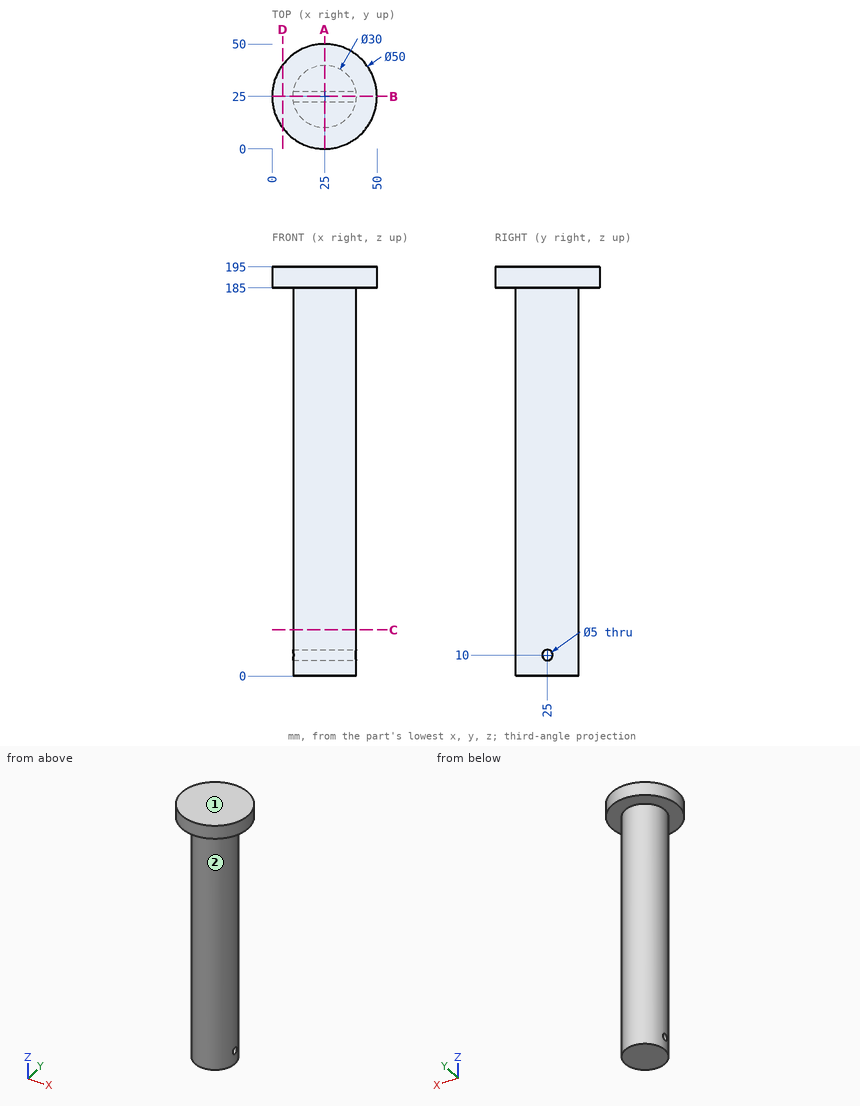
Check sheet for the drawn part. Datum: minimum x, y, z corner. Units: mm. Coordinates: 2 decimals unless noted, no trailing zeros. Order: outer loops, then holes, each group sorted by start corner. A loop starts at its lowest first (then second) coordinate and runs counter-clockwise, first axis right, second up. Notation, with made-up numbers: M 48,12 L 81,12 A25 ccw 81,26 Z; hole C 85,-16 d1. An arc over 180 degrees is marked long. One line per question, with ' | ' between items. Start each with the question number.
Item 1: Material ranges on L1, parallel to Z at x = 28.5, y = 25; L2, parallel to Y at x = 25.5, z = 10; L3, parallel to Y at x = 31, z = 10, recorded low to high. Write a range as [from, to].
Item 2: Cross-section at C-C on z = 22. Enter the section's corners in (x, y).
Item 3: Cross-section at A-A on x = 25. Enter the section's corners in (y, z).
Item 4: Draft check along Y on the marked faces 1 and 2. Enter one of: pulls with the +Y half, pulls with the -Y half, needs draft (parallel to the pull), parting line crosses it, or undercut.
Item 5: Cross-section at B-B on y = 25. Enter the section's corners in (x, z).
Item 6: Gauge pin test, flat ends, axial feed: pin 1 (6 mm diameter, centred on y = 41.5, z = 120.5, fed in from +X); pin 2 (2 mm diameter, centred on x = 21, z = 22, fed in from -Y); pin 3 (10 mm diameter, centred on y = 24.5, z = 28.5, fed in from +X); pin 4 (6 mm diameter, centred on x = 9, y = 23.5, fed in from -Z). Record the tip position at first contact, or that the pin passes through.
Item 7: Cross-section at D-D on x = 5. Enter the section's corners in (y, z).
Findings:
1) L1: z = [0, 7.5], [12.5, 195] | L2: y = [10.01, 22.5], [27.5, 39.99] | L3: y = [11.25, 22.5], [27.5, 38.75]
2) outline: C 25,25 d30
3) outline: M 0,185 L 10,185 L 10,0 L 40,0 L 40,185 L 50,185 L 50,195 L 0,195 Z; hole C 25,10 d5
4) face 1: needs draft | face 2: parting line crosses it
5) outline: M 0,185 L 10,185 L 10,12.5 L 40,12.5 L 40,185 L 50,185 L 50,195 L 0,195 Z; M 10,0 L 40,0 L 40,7.5 L 10,7.5 Z
6) pin 1: stops at x = 31.54 | pin 2: stops at y = 10.3 | pin 3: stops at x = 40 | pin 4: stops at z = 0
7) outline: M 10,185 L 40,185 L 40,195 L 10,195 Z
